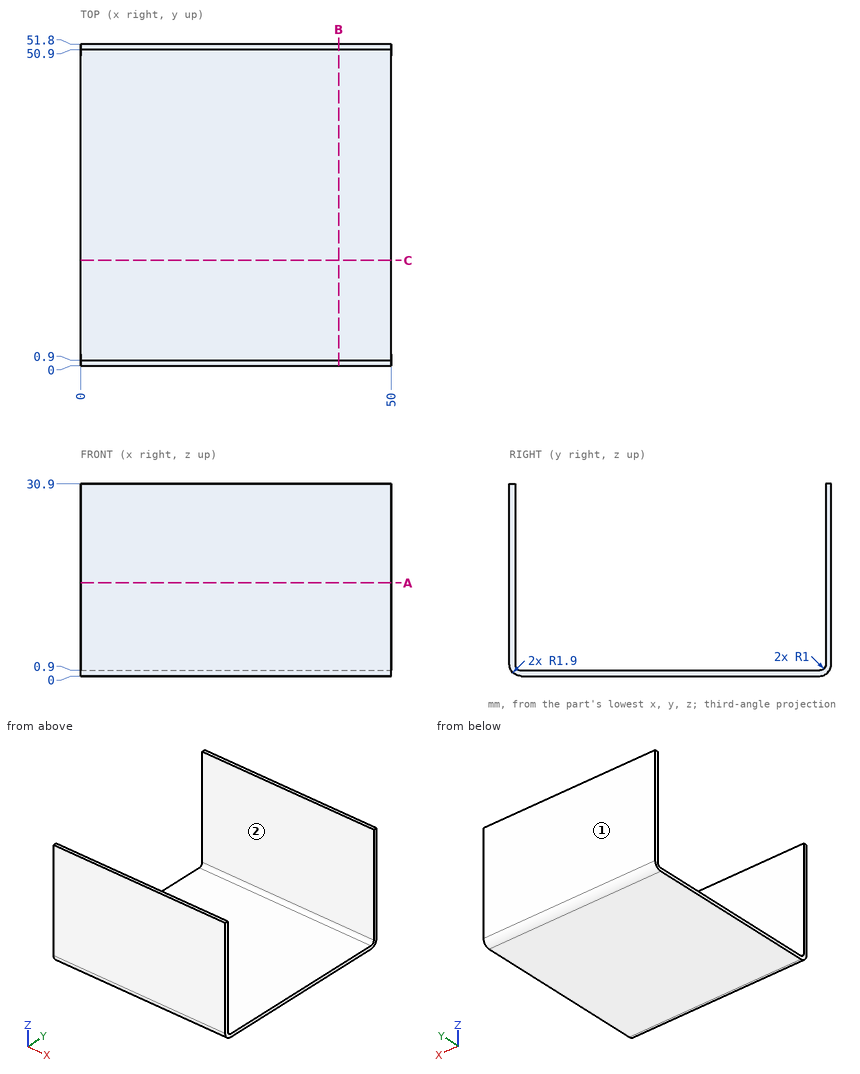
Job drawing, mm, ordinate dimensions from the low corner. One solid piece. A direction names the side the tool comes from. Round coordinates to 2 decimals unless told otherwise and drop trailing zeros. Write each loop counter-clockwise with the first axis right and the second up, starting at its lowest first coordinate (ties: lowest second). Pieces come first, ordered by that corner, then holes. Notation, with made-up numbers: M -7.5,26 L 2.5,26 A15 cw 2.5,45 Z; hole C -34.75,75.25 d3. An arc over 180 degrees is marked long. Return JSON: item names as keys, results as strings. Group by question number.
(1) Drill centre lines: probe 1 along Y at (x, z) = (34.5, 17.5); probe 2 along Z at (x, y) = (25.5, 39). Where is each one in solid material? Low to high.
(2) Saw through at C-C on y = 17. Write the cut outline in (x, z).
(3) Which spindle directions (+Z, -Z, +X, -X, +Y, -Y) get a long thin tool onto all of the face, cutting with end or side? Do the marked faces 1 and 2. Say none if no direction does.
(4) Saw through at A-A on z = 15. Write the cut outline in (x, y), then the cut area to 3 significant figures.
(5) Saw through at B-B on x = 41.5. Write the cut outline in (y, z).
Returned:
{
 "1": {"probe 1": "0 to 0.9, 50.9 to 51.8", "probe 2": "0 to 0.9"},
 "2": {"outline": "M 0,0 L 50,0 L 50,0.9 L 0,0.9 Z"},
 "3": {"face 1": "+Z, -Z, +X, -X, +Y", "face 2": "+Z, +X, -X"},
 "4": {"outline": "M 0,0 L 50,0 L 50,0.9 L 0,0.9 Z; M 0,50.9 L 50,50.9 L 50,51.8 L 0,51.8 Z", "area": "90.0 mm²"},
 "5": {"outline": "M 0,1.9 A1.9 ccw 1.9,0 L 49.9,0 A1.9 ccw 51.8,1.9 L 51.8,30.9 L 50.9,30.9 L 50.9,1.9 A1 cw 49.9,0.9 L 1.9,0.9 A1 cw 0.9,1.9 L 0.9,30.9 L 0,30.9 Z"}
}
